Autodesk Inventor part; units mm, degrees
ref_plane "YZ Plane" through (0, 0, 0) normal (1, 0, 0) x (0, 1, 0)
ref_plane "XZ Plane" through (0, 0, 0) normal (0, 1, 0) x (-1, 0, 0)
ref_plane "XY Plane" through (0, 0, 0) normal (0, 0, 1) x (1, 0, 0)
sketch "Sketch1" plane through (0, 0, 0) normal (0, 1, 0) x (-1, 0, 0)
  line L0 (-4.8, -5.8) -> (0.1217, -5.8)
  line L1 (4.8, -3.25) -> (4.8, 3.25)
  line L2 (0.2433, 5.8) -> (-4.8, 5.8)
  line L3 (-4.8, 5.8) -> (-4.8, -5.8)
  line L4 (-4.8, -5.8) -> (4.8, 5.8) construction
  line L5 (4.8, -5.8) -> (-4.8, 5.8) construction
  line L6 (4.8, 0) -> (4.8, 3.25) construction
  arc A0 (4.8, 3.25) -> (0, 5.8) centre (0.1217, 0.2363) ccw
  line L7 (4.8, 0) -> (4.8, -3.25) construction
  arc A1 (0, -5.8) -> (4.8, -3.25) centre (0.0608, -0.1218) ccw
  circle A2 centre (0, 3.94) radius 1.5
  circle A3 centre (0, 0.08) radius 1.5
  circle A4 centre (0, -3.78) radius 1.5
  arc A5 (-4.8, 4.3) -> (-4.8, 5.3) centre (-4.8, 4.8) ccw
  arc A6 (-4.8, 2.38) -> (-4.8, 3.38) centre (-4.8, 2.88) ccw
  arc A7 (-4.8, 0.46) -> (-4.8, 1.46) centre (-4.8, 0.96) ccw
  arc A8 (-4.8, -1.46) -> (-4.8, -0.46) centre (-4.8, -0.96) ccw
  arc A9 (-4.8, -3.38) -> (-4.8, -2.38) centre (-4.8, -2.88) ccw
  arc A10 (-4.8, -5.3) -> (-4.8, -4.3) centre (-4.8, -4.8) ccw
  line L8 (-4.8, 3.38) -> (-4.8, 2.38)
  line L9 (-4.8, 1.46) -> (-4.8, 0.46)
  line L10 (-4.8, -0.46) -> (-4.8, -1.46)
  line L11 (-4.8, -2.38) -> (-4.8, -3.38)
  line L12 (-4.8, -4.3) -> (-4.8, -5.3)
  point P0 (0, 0)
  dimension "d0" = 9.6
  dimension "d1" = 11.6
  dimension "d2" = 3.25
  dimension "d3" = 3.25
  dimension "d4" = 3
  dimension "d5" = 1.86
  dimension "d8" = 3.86
  dimension "d13" = 1
  dimension "d14" = 1
  dimension "d17" = 1.92
  dimension "d32" = 4.8
extrude "Extrusion2" add sketch "Sketch1" along normal blind 1.75 contours L3 A10 A9 A8 A7 A6 A5 L2 A0 L1 A1 L0
sketch "Sketch2" plane through (0, 1.75, 0) normal (0, 1, 0) x (1, 0, 0)
  line L0 (-1.7477, -2.7588) -> (-2.9764, -3.6192)
  line L1 (-2.9764, -3.6192) -> (-4.4104, -1.5713)
  line L2 (-4.4104, -1.5713) -> (-3.1816, -0.7109)
  line L3 (-3.1816, -0.7109) -> (-1.7477, -2.7588)
  line L4 (-4.55, -1.3) -> (-2.55, -4.3) construction
  line L5 (-2.55, -1.3) -> (-4.55, -4.3) construction
  line L6 (-0.2433, -5.8) -> (4.8, -5.8)
  line L7 (0, -5.8) -> (0, 5.8)
  line L8 (4.8, 5.8) -> (-0.1217, 5.8)
  line L9 (-4.8, 3.25) -> (-4.8, -3.25)
  line L10 (-4.8, 0) -> (4.8, 0) construction
  line L11 (-1.7477, 2.7588) -> (-2.9764, 3.6192)
  line L12 (-2.9764, 3.6192) -> (-4.4104, 1.5713)
  line L13 (-4.4104, 1.5713) -> (-3.1816, 0.7109)
  line L14 (-3.1816, 0.7109) -> (-1.7477, 2.7588)
  point P0 (0, 0)
  point P1 (-3.55, -2.8)
  point P2 (-3.55, -2.8)
  dimension "d26" = 1.5
  dimension "d27" = 2.5
  dimension "d28" = 1.25
  dimension "d29" = 3
extrude "Extrusion3" add sketch "Sketch2" along normal blind 1.5
properties part number "Encoder_optico"
Verification items for the finished model (mm, model axes). A direction names the side the tool comes from. Give positions to 0.01 mm unless a question says otherwise; leave off trailing zeros. Write each loop counter-clockwise with the first axis right and the second up, starting at its lowest first coordinate (ties: lowest second). Pieces come first, ordered by that corner, then holes.
(1) Material ranges on line 1 (Z direction, x = 0, y = 0.55); line 2 (Y direction, x = 3.25, z = -4.5); line 3 (X direction, y = 0.55, z = 4.25), recorded low to high.
(2) Cross-section at A-A (y = 1.05). Enter the section's corners in (x, z), plus the area to 3 significant figures.
(3) Cross-section at D-D (x = -1). Enter the section's corners in (y, z).
(4) Mould release check, pull along Z, two halves, no side actions. Record for faces 6 (the face through (1.19, 0.86, 0.99)), 7 (the face through (-3.683, 2.49, -2.61)), 8 (the face through (4.8, 1, -2)): +Z half, -Z half, draft (parallel to the pull), parting line (faces both ways), or undercut.
(5) Access from +Z, -Z, +X, -X, +Y, -Y to the whole of each face (thin tool, end or side, straight path). Record for faces 1 (the face through (-2.35, 2.49, -3.18)), 2 (the face through (-2.35, 2.49, 3.18)), 3 (the face through (-3.805, 2.49, 1.147)), 4 (the face through (-3.683, 2.49, 2.61)), 5 (the face through (-2.475, 2.49, -1.721)).
(6) Cross-section at C-C (y = 2.45). Enter the section's corners in (x, z).
(7) Gauge pin test, flat end, axial feed: pin 1 (3.5 mm diameter, centred on x = 0, z = 3.94, fed in from +Y). Record the tip position at first contact, or that the pin passes through.
(8) Cross-section at B-B (z = 0.08). Enter the section's corners in (x, y), plus the area to 4 significant figures.
Worked out:
1. line 1: z = -5.8 to -5.28, -2.28 to -1.42, 1.58 to 2.44, 5.44 to 5.8
1. line 2: y = 0 to 1.75
1. line 3: x = -3.98 to -1.47, 1.47 to 4.8
2. outline: (-4.8, -3.25) arc R5.68 ccw to (-0.12, -5.8) - (4.8, -5.8) - (4.8, -5.3) arc R0.5 cw to (4.8, -4.3) - (4.8, -3.38) arc R0.5 cw to (4.8, -2.38) - (4.8, -1.46) arc R0.5 cw to (4.8, -0.46) - (4.8, 0.46) arc R0.5 cw to (4.8, 1.46) - (4.8, 2.38) arc R0.5 cw to (4.8, 3.38) - (4.8, 4.3) arc R0.5 cw to (4.8, 5.3) - (4.8, 5.8) - (-0.24, 5.8) arc R5.57 ccw to (-4.8, 3.25) - close; hole circle Ø3 at (0, -3.78); hole circle Ø3 at (0, 0.08); hole circle Ø3 at (0, 3.94)
2. area: 80.7 mm2
3. outline: (0, -5.72) - (1.75, -5.72) - (1.75, -4.9) - (0, -4.9) - close; (0, -2.66) - (1.75, -2.66) - (1.75, -1.04) - (0, -1.04) - close; (0, 1.2) - (1.75, 1.2) - (1.75, 2.82) - (0, 2.82) - close; (0, 5.06) - (1.75, 5.06) - (1.75, 5.73) - (0, 5.73) - close
4. face 6: undercut
4. face 7: -Z half
4. face 8: draft
5. face 1: -Z, +X, +Y
5. face 2: +Z, +X, +Y
5. face 3: -X, +Y
5. face 4: +Z, -X, +Y
5. face 5: +X, +Y
6. outline: (-4.41, -1.57) - (-2.98, -3.62) - (-1.75, -2.76) - (-3.18, -0.71) - close; (-4.41, 1.57) - (-3.18, 0.71) - (-1.75, 2.76) - (-2.98, 3.62) - close
7. pin 1: stops at y = 1.75
8. outline: (-4.8, 0) - (-1.5, 0) - (-1.5, 1.75) - (-4.8, 1.75) - close; (1.5, 0) - (4.8, 0) - (4.8, 1.75) - (1.5, 1.75) - close
8. area: 11.55 mm2
